Here's how the part is built. I have some questions about the finished solid (model axes, mm). A direction names the side the tool comes from. Give positions to 0.01 mm unless a question says otherwise; leave off trailing zeros. Write each loop counter-clockwise with the first axis right and the second up, starting at its lowest first coordinate (ties: lowest second). Pieces come first, ordered by that corner, then holes. Notation, with made-up numbers: (83, 23) - (132, 23) arc R20 ccw to (132, 61) - close; hole circle Ø7 at (58, -11). An arc over 180 degrees is marked (long way). Use a Markdown table: item, result.
```python
from build123d import *

# Parameters (mm, degrees)
SKETCH1_W           = 40
SKETCH1_H           = 40
BOSS_EXTRUDE1_DEPTH = 5
SKETCH3_R           = 1.4
CUT_EXTRUDE1_DEPTH  = 10
SKETCH4_R           = 5.75
BOSS_EXTRUDE2_DEPTH = 45
CHAMFER1_SIZE       = 6
SKETCH6_R           = 1.4
CUT_EXTRUDE2_DEPTH  = 16
FILLET1_R           = 1


with BuildPart() as part:
    # Sketch1 → Boss-Extrude1 (new body)
    with BuildSketch(Plane(origin=(0, 0, 0), x_dir=(1, 0, 0), z_dir=(0, 1, 0))):
        Rectangle(SKETCH1_W, SKETCH1_H)
    extrude(amount=BOSS_EXTRUDE1_DEPTH)

    # Sketch3 → Cut-Extrude1 (cut)
    with BuildSketch(Plane.XZ):
        with Locations(Location((-16.5, -16.5, 0), (0, 0, 270))):
            Circle(SKETCH3_R)
        with Locations(Location((-16.5, 16.5, 0), (0, 0, 270))):
            Circle(SKETCH3_R)
        with Locations(Location((16.5, 16.5, 0), (0, 0, 270))):
            Circle(SKETCH3_R)
        with Locations(Location((16.5, -16.5, 0), (0, 0, 270))):
            Circle(SKETCH3_R)
    extrude(amount=-CUT_EXTRUDE1_DEPTH, mode=Mode.SUBTRACT)

    # Sketch4 → Boss-Extrude2 (add)
    with BuildSketch(Plane(origin=(0, 5, 0), x_dir=(1, 0, 0), z_dir=(0, 1, 0))):
        with Locations(Location((0, 0, 0), (0, 0, 90))):
            Circle(SKETCH4_R)
    extrude(amount=BOSS_EXTRUDE2_DEPTH)

    # Chamfer1
    chamfer1_edges = [part.edges().sort_by_distance(p)[0] for p in [
        (0, 5, 5.75),
    ]]
    chamfer(chamfer1_edges, length=CHAMFER1_SIZE)

    # Sketch6 → Cut-Extrude2 (cut)
    with BuildSketch(Plane(origin=(0, 50, 0), x_dir=(1, 0, 0), z_dir=(0, 1, 0))):
        with Locations(Location((0, 0, 0), (0, 0, 270))):
            Circle(SKETCH6_R)
    extrude(amount=-CUT_EXTRUDE2_DEPTH, mode=Mode.SUBTRACT)

    # Fillet1
    fillet1_edges = [part.edges().sort_by_distance(p)[0] for p in [
        (20, 2.5, 20),
        (-20, 2.5, 20),
        (-20, 2.5, -20),
        (20, 2.5, -20),
    ]]
    fillet(fillet1_edges, radius=FILLET1_R)


solid = part.part
```
Item 1: If we section it at C-C, the plane x = 0: Write out the boundary of the cut face in (y, z).
Values:
| item | result |
|---|---|
| outline | (0, -20) - (5, -20) - (5, -11.75) - (11, -5.75) - (50, -5.75) - (50, -1.4) - (34, -1.4) - (34, 1.4) - (50, 1.4) - (50, 5.75) - (11, 5.75) - (5, 11.75) - (5, 20) - (0, 20) - close |
Item 2: If we section it at B-B, the plane x = -16.5: Write out the boundary of the cut face in (y, z), plus the area to 3 significant figures.
Values:
| item | result |
|---|---|
| outline | (0, -20) - (5, -20) - (5, -17.9) - (0, -17.9) - close; (0, -15.1) - (5, -15.1) - (5, 15.1) - (0, 15.1) - close; (0, 17.9) - (5, 17.9) - (5, 20) - (0, 20) - close |
| area | 172 mm2 |
Item 3: If we section it at D-D, the plane y = 19: Write out the boundary of the cut face in (x, z).
Values:
| item | result |
|---|---|
| outline | circle Ø11.5 at (0, 0) |
Item 4: I need wall thicknesses on line 1 along X through (y, z) = (1, 16); line 2 along X through (y, z) = (46.5, 0); line 3 along Y through (x, z) = (-18, -8). Which ranges of each line are inside material? Lowest first, please. Write a range as [from, to].
Values:
| item | result |
|---|---|
| line 1 | x = [-20, -17.81], [-15.19, 15.19], [17.81, 20] |
| line 2 | x = [-5.75, -1.4], [1.4, 5.75] |
| line 3 | y = [0, 5] |
Item 5: Thinking about a two-plate mould opening in Z: for faces 3 (the flat face through (0, 2, 20)), 4 (the flat face through (0, 2, -20)), 5 (the cylindrical face through (17.45, 2.46, 17.53)), 6 (the flat face through (9, 5, -9)), which applies, +Z half, -Z half, draft (parallel to the pull), parting line (faces both ways), or undercut?
Values:
| item | result |
|---|---|
| face 3 | +Z half |
| face 4 | -Z half |
| face 5 | undercut |
| face 6 | draft |
Item 6: Will these pins go through, and if not, where does the flat tip stop? pin 1 Ø2.5 at (x, z) = (16.5, 16.5) entering from +Y; pin 2 Ø1.7 at (x, z) = (0, 0) entering from +Y; pin 3 Ø8 at (y, z) = (9.5, 10.5) entering from -X; pin 4 Ø8 at (x, z) = (-15.5, 2) entering from +Y.
Values:
| item | result |
|---|---|
| pin 1 | passes through |
| pin 2 | stops at y = 34 |
| pin 3 | stops at x = -6.6 |
| pin 4 | stops at y = 5.12 |
Item 7: If we section it at A-A, the plane z = -16.5: Write out the boundary of the cut face in (x, y), plus the area to 3 significant figures.
Values:
| item | result |
|---|---|
| outline | (-20, 0) - (-17.9, 0) - (-17.9, 5) - (-20, 5) - close; (-15.1, 0) - (15.1, 0) - (15.1, 5) - (-15.1, 5) - close; (17.9, 0) - (20, 0) - (20, 5) - (17.9, 5) - close |
| area | 172 mm2 |
Item 8: For faces 1 (the cylindrical face through (17.45, 2.46, -15.47)), 2 (the flat face through (0, 34, 0)), which set-ups out of +Z, -Z, +X, -X, +Y, -Y let a thin tool reach every point of the face, with its end or its side?
Values:
| item | result |
|---|---|
| face 1 | +Y, -Y |
| face 2 | +Y |
